Autodesk Inventor part; units mm, degrees
ref_plane "YZ Plane" through (0, 0, 0) normal (1, 0, 0) x (0, 1, 0)
ref_plane "XZ Plane" through (0, 0, 0) normal (0, 1, 0) x (-1, 0, 0)
ref_plane "XY Plane" through (0, 0, 0) normal (0, 0, 1) x (1, 0, 0)
sketch "Boceto1" plane through (0, 0, 0) normal (0, 1, 0) x (-1, 0, 0)
  line L0 (8.8742, 70.1532) -> (-86.8258, 70.1532)
  line L1 (-86.8258, 70.1532) -> (-86.8258, 20.1532)
  line L2 (-86.8258, 20.1532) -> (8.8742, 20.1532)
  line L3 (8.8742, 20.1532) -> (8.8742, 70.1532)
  dimension "d0" = 95.7
  dimension "d1" = 50
extrude "Extrusión1" add sketch "Boceto1" along normal blind 10
sketch "Boceto2" plane through (86.8258, 0, 70.1532) normal (1, 0, 0) x (0, 0, -1)
  line L0 (0, 0) -> (0, 10)
  line L1 (50, 0) -> (50, 10)
  circle A0 centre (5, 5) radius 2
  circle A1 centre (45, 5) radius 2
  point P0 (70.1532, 0)
  dimension "d4" = 4
  dimension "d5" = 5
  dimension "d6" = 4
  dimension "d7" = 5
sketch "Boceto3" plane through (-8.8742, 0, 20.1532) normal (-1, 0, 0) x (0, 0, 1)
  circle A0 centre (5, 5) radius 2
  line L0 (0, 10) -> (50, 10)
  line L1 (0, 0) -> (0, 10)
  circle A1 centre (45, 5) radius 2
  line L2 (50, 0) -> (50, 10)
  dimension "d8" = 4
  dimension "d9" = 5
  dimension "d10" = 5
  dimension "d11" = 4
  dimension "d12" = 5
  dimension "d13" = 5
hole "Agujero1" at (-8.8742, 5, 25.1532) at (-8.8742, 5, 65.1532) direction (1, 0, 0) diameter 4 depth 10 tip angle 118
hole "Agujero2" at (86.8258, 5, 65.1532) at (86.8258, 5, 25.1532) direction (-1, 0, 0) diameter 4 depth 10 tip angle 118
thread "Rosca1"
thread "Rosca2"
thread "Rosca3"
thread "Rosca4"
sketch "Sketch4" plane through (0, 10, 0) normal (0, 1, 0) x (1, 0, 0)
  circle A0 centre (6.1258, -45.1532) radius 3
  line L0 (-8.8742, -20.1532) -> (-8.8742, -70.1532)
  dimension "d36" = 6
  dimension "d37" = 15
extrude "Extrusion2" cut sketch "Sketch4" against normal blind 10
properties part number "Soporte para Culata Carcasa Izquierdo" material "Aluminio 6061"
The listing builds one solid part. Answer for the finished solid, in the listing's coordinates (mm). A direction names the side the tool comes from. Round coordinates to 2 decimals unless told otherwise and drop trailing zeros. Put each result on its own line as item: value. Start each with the question number.
(1) Determine the mould class of faces 4 (the cylindrical face through (-3.804, 4.912, 63.155)), 5 (the flat face through (-8.874, 5, 45)), 6 (the flat face through (40, 0, 46)) for opening direction Y: released by +Y, released by -Y, zero draft, split by the parting line, or undercut.
(2) Straight lines are drawn through the part: probe 1 along Z at (x, y) = (-1.75, 5); probe 2 along Z at (x, y) = (-1.5, 5.5); probe 3 along X at (y, z) = (7.25, 45). For each, find the intervals that lie inside material, in ascending order. Write a range as from..to.
(3) Given P1, Ø3.5, axis at y = 5, z = 25.15, coming from the +X side; P2, Ø2.5, axis at y = 5, z = 65.15, coming from the -X side, each flat-ended and moving along its own axis, determine where each tip first touches the part or whether it passes through.
(4) For faces 1 (the flat face through (40, 10, 46)), 2 (the cylindrical face through (-3.804, 4.912, 23.155)), 3 (the cylindrical face through (81.756, 5.766, 63.306)), determine the directions among +Z, -Z, +X, -X, +Y, -Y from which every point of the face is accessible in a straight line to the end or side of a thin tool.
Reply:
1. face 4: undercut
1. face 5: zero draft
1. face 6: released by -Y
2. probe 1: 20.15..23.15, 27.15..63.15, 67.15..70.15
2. probe 2: 20.15..23.22, 27.09..63.22, 67.09..70.15
2. probe 3: -8.87..3.13, 9.12..86.83
3. P1: x = 76.68
3. P2: x = 1.57
4. face 1: +Z, -Z, +X, -X, +Y
4. face 2: -X
4. face 3: +X
